Verification items for the finished model (mm, model axes). Face numbers are marked on the shaded views. A direction names the side the tool comes from. Give positions to 0.01 mm unless a question says otherwise; leave off trailing zeros. Order: outer loops, then holes, each group sorted by start corner. A loop starts at its lowest first (then second) coordinate and runs counter-clockwise, first axis right, second up. Notation, with made-up numbers: (-19.5, 40) - (14.5, 40) arc R8 ccw to (14.5, 55) - close; hole circle Ø6 at (40, 67). An arc over 180 degrees is marked (long way). Answer as a JSON object with one key per item and string values. Group by question number.
(1) Section check B-B (x = -5.15). Record the boundary of the cut face in (y, z).
(2) Section check D-D (x = -1.5). Record the boundary of the cut face in (y, z), then the cut area to 3 significant figures.
(3) Section check A-A (y = 0). Record the boundary of the cut face in (x, z).
(4) Access from +Z, -Z, +X, -X, +Y, -Y to the whole of each face (thin tool, end or side, straight path). Record for the marked faces 1, 2, 3 and 4.
(5) Depth check by flat-ended pin: pin 1 Ø1 at (x, y) = (-5.5, -0.5) entering from -Z; pin 2 Ø0.6 at (x, y) = (-7.5, 0.5) entering from +Z; pin 3 Ø2 at (y, z) = (2.5, 2) entering from +X. Enter the tip coordinate at first touch or a pass-through.
(6) Section check C-C (z = 0.75). Record the boundary of the cut face in (x, y), then the cut area to 3 significant figures.
(7) Thickness scan on line 1 (X direction, y = -1.5, z = 3.25); line 2 (Y direction, x = -5.15, z = -6.35); line 3 (Z direction, x = -6, y = -5). Record the ranges inside material, lowest first.
```python
from build123d import *

# Parameters (mm, degrees)
F1_DEPTH       = 6.25
F2_W           = 2
F2_H           = 4.5
F3_DEPTH       = 10.401
F5_D           = 2
F5_DEPTH       = 38
F5_CBORE_D     = 3.5
F5_CBORE_DEPTH = 3
F5_TIP         = 0.600860619


with BuildPart() as f1:
    # F0 (on Front) → F1 (new body, symmetric)
    with BuildSketch(Plane.XZ):
        Polygon((17, -3.5), (0, 0), (0, 4.5), (-4.25, 4.5), (-4.25, -2.75), (-6.25, -2.75), (-6.25, 4.5), (-10.4, 4.5), (-10.4, -8), (17, -8), align=None)
    extrude(amount=F1_DEPTH, both=True)

    # F2 (on Right) → F3 (cut, through all)
    with BuildSketch(Plane.YZ):
        with Locations((0, 2.25)):
            Rectangle(F2_W, F2_H)
    extrude(amount=-F3_DEPTH, mode=Mode.SUBTRACT)

    # F5
    with Locations(Plane(origin=(0, 0, -8), x_dir=(1, 0, 0), z_dir=(0, 0, -1))):
        with Locations((-5.15, 0)):
            CounterBoreHole(F5_D / 2, F5_CBORE_D / 2, F5_CBORE_DEPTH, depth=F5_DEPTH)
            with Locations((0, 0, -(F5_DEPTH + F5_TIP / 2))):  # 118° drill point
                Cone(0, F5_D / 2, F5_TIP, mode=Mode.SUBTRACT)


solid = f1.part
```
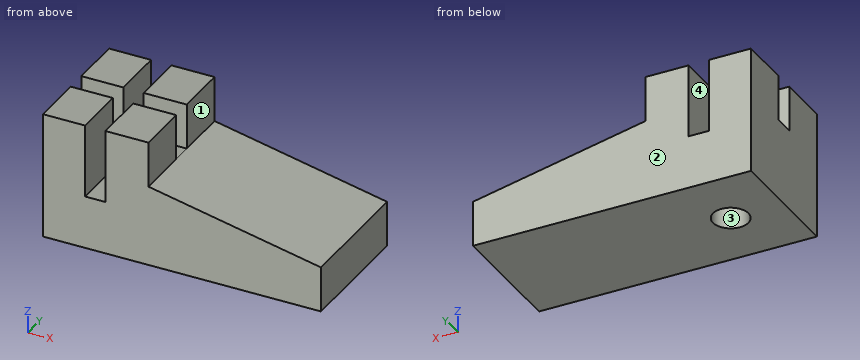
Solutions:
{
 "1": {"outline": "(-6.25, -8) - (-1.75, -8) - (-1.75, -5) - (-1, -5) - (-1, -2.75) - (-6.25, -2.75) - close; (1, -5) - (1.75, -5) - (1.75, -8) - (6.25, -8) - (6.25, -2.75) - (1, -2.75) - close"},
 "2": {"outline": "(-6.25, -8) - (6.25, -8) - (6.25, 4.5) - (1, 4.5) - (1, 0) - (-1, 0) - (-1, 4.5) - (-6.25, 4.5) - close", "area": "147 mm2"},
 "3": {"outline": "(-10.4, -8) - (-6.9, -8) - (-6.9, -5) - (-6.15, -5) - (-6.15, -2.75) - (-6.25, -2.75) - (-6.25, 0) - (-10.4, 0) - close; (-4.15, -5) - (-3.4, -5) - (-3.4, -8) - (17, -8) - (17, -3.5) - (0, 0) - (-4.15, 0) - close"},
 "4": {"face 1": "+Z, +X, +Y, -Y", "face 2": "+Z, -Z, +X, -X, +Y", "face 3": "-Z", "face 4": "+Z, +Y, -Y"},
 "5": {"pin 1": "stops at z = -5", "pin 2": "stops at z = 0", "pin 3": "stops at x = 0"},
 "6": {"outline": "(-10.4, -6.25) - (-6.25, -6.25) - (-6.25, -1) - (-10.4, -1) - close; (-10.4, 1) - (-6.25, 1) - (-6.25, 6.25) - (-10.4, 6.25) - close; (-4.25, -6.25) - (0, -6.25) - (0, -1) - (-4.25, -1) - close; (-4.25, 1) - (0, 1) - (0, 6.25) - (-4.25, 6.25) - close", "area": "88.2 mm2"},
 "7": {"line 1": "x = -10.4 to -6.25, -4.25 to 0", "line 2": "y = -6.25 to -1.75, 1.75 to 6.25", "line 3": "z = -8 to -2.75"}
}
